Geometry check sheet. Reference: drawing and pictorial views, mm from the part's lowest x, y, z. A direction names the side the tool comes from. Give positions to 0.01 mm unless a question says otherwise; leave off trailing zeros. Write each loop counter-clockwise with the first axis right and the second up, starting at its lowest first coordinate (ties: lowest second). Pieces come first, ordered by that corner, then holes. Notation, with made-up numbers: (-11.75, 85.5) - (29.25, 85.5) arc R18 ccw to (29.25, 90.5) - close; hole circle Ø9 at (73, 36.5). An arc over 180 degrees is marked (long way). Write item = value, one per line. Start each with the question number.
(1) Draft check along Y on the marked faces 3, 4, 5 and 6. Enter one of: pulls with the +Y half, pulls with the -Y half, needs draft (parallel to the pull), parting line crosses it, or undercut.
(2) Access from +Z, -Z, +X, -X, +Y, -Y to the whole of each face (thin tool, end or side, straight path). Record for the marked faces 1 and 2.
(3) Section check C-C, the plane z = 2.05. Enter the section's corners in (x, y), plus the area to 3 significant figures.
(4) Section check A-A, the plane x = 6.5. Enter the section's corners in (y, z), plus the area to 3 significant figures.
(5) Thickness scan on L1, parallel to Y at x = 14.25, z = 0.9. Record the ranges inside material, lowest first.
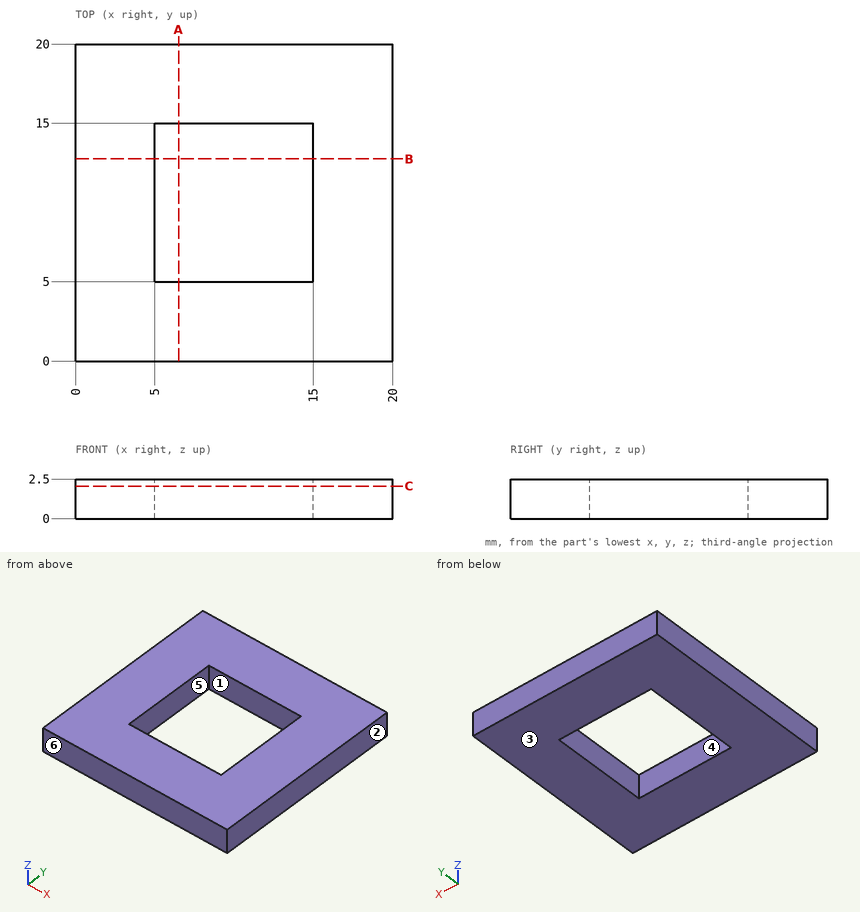
Model answer:
q1.face_3 = needs draft
q1.face_4 = undercut
q1.face_5 = undercut
q1.face_6 = pulls with the -Y half
q2.face_1 = +Z, -Z
q2.face_2 = +Z, -Z, +X, +Y, -Y
q3.outline = (0, 0) - (20, 0) - (20, 20) - (0, 20) - close; hole (5, 5) - (15, 5) - (15, 15) - (5, 15) - close
q3.area = 300 mm²
q4.outline = (0, 0) - (5, 0) - (5, 2.5) - (0, 2.5) - close; (15, 0) - (20, 0) - (20, 2.5) - (15, 2.5) - close
q4.area = 25.0 mm²
q5.L1 = 0 to 5, 15 to 20
